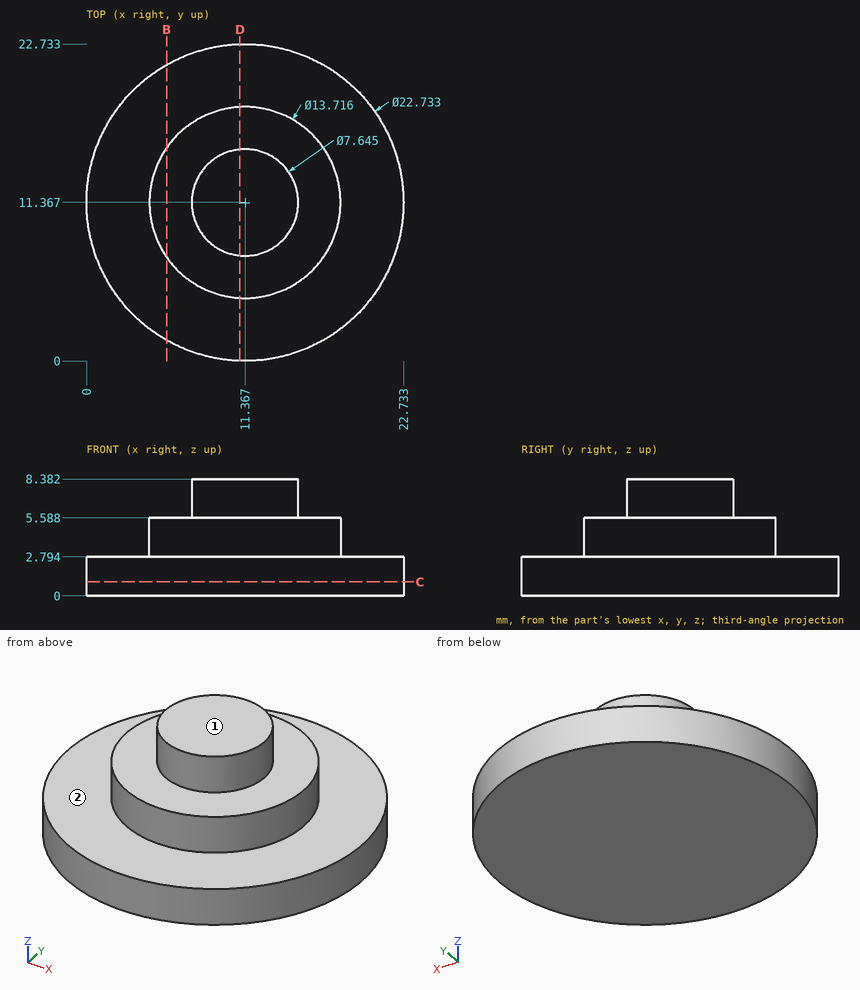
Geometry check sheet. Reference: drawing and pictorial views, mm from the part's lowest x, y, z. A direction names the side the tool comes from. Give positions to 0.01 mm unless a question says otherwise; leave off trailing zeros. Order: outer loops, then holes, each group sorted by start corner. A loop starts at its lowest first (then second) coordinate and runs counter-clockwise, first axis right, second up. Notation, with made-up numbers: M -11,14 L 34,14 A18 cw 34,30 Z; hole C 5.25,59.25 d1. An arc over 180 degrees is marked long. Answer as CSV lines item,"result". Start each with the question number.
Item 1: Gauge pin test, flat ends, axial feed: P1, Ø1.5, axis at y = 17, z = 5.5, coming from the -X side; P2, Ø2, axis at y = 16, z = 2, coming from the -X side; P3, Ø3, axis at x = 14.5, z = 4.5, coming from the -Y side (1 decimal). Record the tip position at first contact, or that the pin passes through.
Item 2: Cross-section at B-B on x = 5.75. Enter the section's corners in (y, z) (1 decimal).
Item 3: Cross-section at D-D on x = 11. Enter the section's corners in (y, z) (1 decimal), plus the area to 3 significant figures.
Item 4: Thickness scan on line 1 (Z direction, x = 4, y = 17) (1 decimal); line 2 (X direction, y = 11.25, z = 3.5); line 3 (Z direction, x = 16.5, y = 10). Record the ranges inside material, lowest first. Write a range as [from, to].
Item 5: Cross-section at C-C on z = 1. Enter the section's corners in (x, y), plus the area to 3 significant figures.
Item 6: Tool access check on the marked faces 1 and 2. Record the directions out of +Z, -Z, +X, -X, +Y, -Y that give a thin tool (end or side, any length) a straight path to the whole face; none if there is none.
Established:
1,P1,"stops at x = 6.55"
1,P2,"stops at x = 0.6"
1,P3,"stops at y = 4.7"
2,outline,"M 1.5,0 L 21.2,0 L 21.2,2.8 L 15.3,2.8 L 15.3,5.6 L 7.4,5.6 L 7.4,2.8 L 1.5,2.8 Z"
3,outline,"M 0,0 L 22.7,0 L 22.7,2.8 L 18.2,2.8 L 18.2,5.6 L 15.2,5.6 L 15.2,8.4 L 7.6,8.4 L 7.6,5.6 L 4.5,5.6 L 4.5,2.8 L 0,2.8 Z"
3,area,"123 mm^2"
4,line 1,"z = [0, 2.8]"
4,line 2,"x = [4.51, 18.22]"
4,line 3,"z = [0, 5.59]"
5,outline,"C 11.37,11.37 d22.73"
5,area,"406 mm^2"
6,face 1,"+Z, +X, -X, +Y, -Y"
6,face 2,"+Z"
